Design review of the part shown in the three views and the two pictorial views. Dimensions are in mm from the part's minimum x, y and z. Give positions to 0.01 mm unless a question says otherwise; leave off trailing zeros. Loops run counter-clockwise (first coordinate to the right, second up) from the corner with the lowest first, then second, coordinate; pieces in that order, holes last. Notation, with made-up numbers: (82.5, 20) - (101.5, 20) arc R13 ccw to (101.5, 28) - close; hole circle Ø8 at (31.5, 22). An arc over 180 degrees is marked (long way). Answer as a JSON object with one key per item and string values.
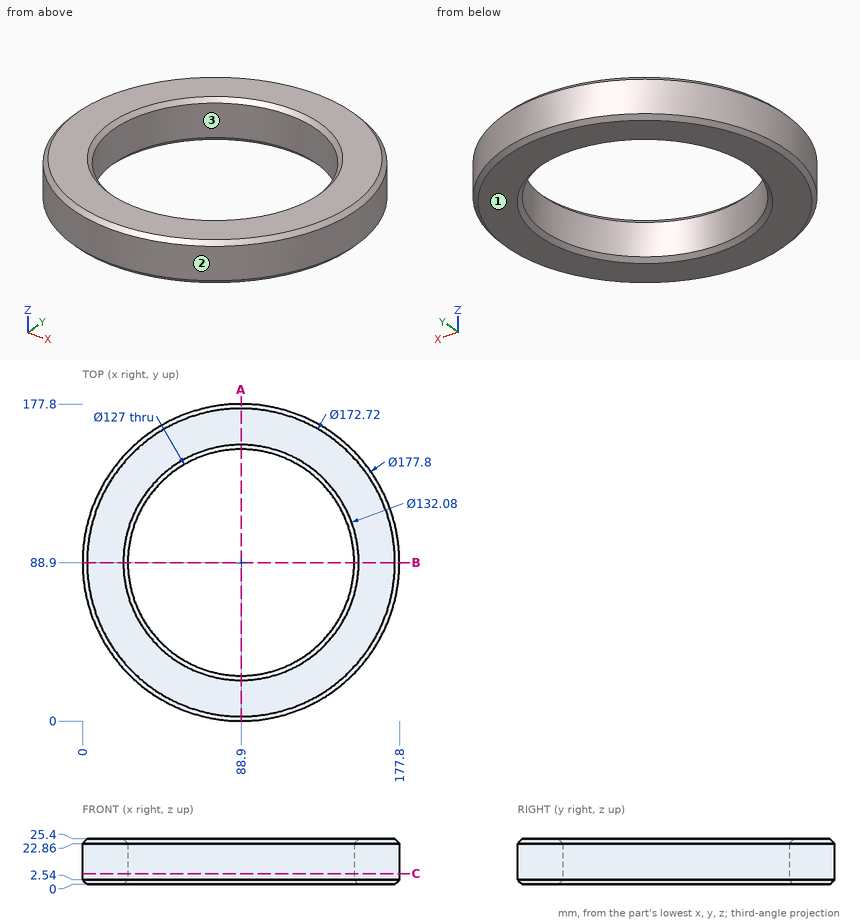
Q1. To check wall thickness, follow probe 1 along Y at (x, z) = (88.9, 14.5); probe 2 along X at (y, z) = (92.5, 7.25); probe 3 along Y at (x, z) = (31.5, 3.5). State the ranges of each line that lie inside material, in increasing order. Write a range as [from, to].
Results:
{"probe 1": "y = [0, 25.4], [152.4, 177.8]", "probe 2": "x = [0.07, 25.5], [152.3, 177.73]", "probe 3": "y = [21.01, 61.74], [116.06, 156.79]"}
Q2. Clearance check with flat-ended pins moving along their axes: pin 1 Ø1 at (y, z) = (47.5, 11.5) entering from -X; pin 2 Ø6 at (x, z) = (65.5, 19) entering from +Y; pin 3 Ø1.5 at (x, z) = (148, 21) entering from +Y. State where each tip first meets the part, or that it passes through.
Results:
{"pin 1": "stops at x = 9.97", "pin 2": "stops at y = 175.43", "pin 3": "stops at y = 155.97"}
Q3. Consider section A-A, the plane x = 88.9. State the section outline as (y, z) points, plus the area to 3 significant figures.
Results:
{"outline": "(0, 2.54) - (2.54, 0) - (22.86, 0) - (25.4, 2.54) - (25.4, 22.86) - (22.86, 25.4) - (2.54, 25.4) - (0, 22.86) - close; (152.4, 2.54) - (154.94, 0) - (175.26, 0) - (177.8, 2.54) - (177.8, 22.86) - (175.26, 25.4) - (154.94, 25.4) - (152.4, 22.86) - close", "area": "1,260 mm^2"}
Q4. Consider section C-C, the plane z = 6. State the section outline as (x, y) points.
Results:
{"outline": "circle Ø177.8 at (88.9, 88.9); hole circle Ø127 at (88.9, 88.9)"}
Q5. The part is to be moulded in two halves that separate along Y. For the marked faces 1, 2 and 3, say which applies: +Y half, -Y half, draft (parallel to the pull), parting line (faces both ways), or undercut.
Results:
{"face 1": "draft", "face 2": "parting line", "face 3": "undercut"}
